```python
from build123d import *

# Parameters (mm, degrees)
F1_DEPTH     = 10.16
F5_R         = 1.4478
F6_DEPTH     = 25.4
F10_DEPTH    = 1.27
F11_T1_DEPTH = 22.6859947386
F11_T4_ANGLE = 28.0699881424
F11_T6_ANGLE = 28.0699881424


# Not quite as in the source:
# - a fillet or chamfer that OpenCascade refuses, or shapes differently, is made with other operations: its cross-section is extruded or revolved along the edge and cut away or added


with BuildPart() as f1:
    # F0 (on Top) → F1 (new body)
    with BuildSketch(Plane.XY):
        with BuildLine():
            ThreePointArc((0, 95.25), (-8.3015844967, 94.8875449932), (-16.5399889228, 93.8029384744))
            Line((-16.5399889228, 93.8029384744), (-15.6578561802, 88.8001150891))
            ThreePointArc((-15.6578561802, 88.8001150891), (-7.8588333236, 89.8268759269), (0, 90.17))
            Line((0, 90.17), (0, 95.25))
        make_face()
        with BuildLine():
            Line((15.6578561802, 88.8001150891), (16.5399889228, 93.8029384744))
            ThreePointArc((16.5399889228, 93.8029384744), (8.3015844967, 94.8875449932), (0, 95.25))
            Line((0, 95.25), (0, 90.17))
            ThreePointArc((0, 90.17), (7.8588333236, 89.8268759269), (15.6578561802, 88.8001150891))
        make_face()
    extrude(amount=F1_DEPTH)

    # F5 (on line) → F6 (cut)
    with BuildSketch(Plane(origin=(0, 95.25, 0), x_dir=(-1, 0, 0), z_dir=(0, 1, 0))):
        with Locations((-9.525, 5.08)):
            Circle(F5_R)
        with BuildLine():
            ThreePointArc((10.9728, 5.08), (9.525, 6.5278), (8.0772, 5.08))
            ThreePointArc((8.0772, 5.08), (9.525, 3.6322), (10.9728, 5.08))
        make_face()
    extrude(amount=-F6_DEPTH, mode=Mode.SUBTRACT)

    # F9 (on line) → F10 (cut, symmetric)
    with BuildSketch(Plane(origin=(0, 90.17, 0), x_dir=(-1, 0, 0), z_dir=(0, 1, 0))):
        Polygon((7.62, 8.3795567884), (5.715, 5.08), (7.62, 1.7804432116), (11.43, 1.7804432116), (13.335, 5.08), (11.43, 8.3795567884), align=None)
        Polygon((-11.43, 8.3795567884), (-13.335, 5.08), (-11.43, 1.7804432116), (-7.62, 1.7804432116), (-5.715, 5.08), (-7.62, 8.3795567884), align=None)
    extrude(amount=F10_DEPTH, both=True, mode=Mode.SUBTRACT)

    # F11: fillet of radius 2.54 on 4 edges, made by hand

    # F11_s2 → F11_t1 (cut)
    with BuildSketch(Plane.XY.offset(-6.2629973693)):
        with BuildLine():
            ThreePointArc((13.2190987409, 89.1957640725), (15.0767198196, 89.6478290697), (16.0928794122, 91.2672544357))
            Line((16.0928794122, 91.2672544357), (15.6578561802, 88.8001150891))
            ThreePointArc((15.6578561802, 88.8001150891), (14.4398326136, 89.0062926657), (13.2190987409, 89.1957640725))
        make_face()
        with BuildLine():
            ThreePointArc((-16.0928794122, 91.2672544357), (-15.0767198196, 89.6478290697), (-13.2190987409, 89.1957640725))
            ThreePointArc((-13.2190987409, 89.1957640725), (-14.4398326136, 89.0062926657), (-15.6578561802, 88.8001150891))
            Line((-15.6578561802, 88.8001150891), (-16.0928794122, 91.2672544357))
        make_face()
    extrude(amount=F11_T1_DEPTH, mode=Mode.SUBTRACT)

    # F11_s3 → F11_t4 (revolve, cut)
    with BuildSketch(Plane(origin=(0, 0, 0), x_dir=(0, 0, 1), z_dir=(-0.9701477887, -0.24251447, 0))):
        with BuildLine():
            ThreePointArc((7.62, 90.17), (9.4160512242, 90.9139487758), (10.16, 92.71))
            Line((10.16, 92.71), (10.16, 90.17))
            Line((10.16, 90.17), (7.62, 90.17))
        make_face()
    revolve(axis=Axis((0, 0, 10.16), (0, 0, -1)), revolution_arc=F11_T4_ANGLE, mode=Mode.SUBTRACT)

    # F11_s5 → F11_t6 (revolve, cut)
    with BuildSketch(Plane(origin=(0, 0, 0), x_dir=(0, 0, 1), z_dir=(-0.9701477887, -0.24251447, 0))):
        with BuildLine():
            ThreePointArc((2.54, 90.17), (0.7439487758, 90.9139487758), (0, 92.71))
            Line((0, 92.71), (0, 90.17))
            Line((0, 90.17), (2.54, 90.17))
        make_face()
    revolve(axis=Axis((0, 0, 0), (0, 0, -1)), revolution_arc=F11_T6_ANGLE, mode=Mode.SUBTRACT)


solid = f1.part
```
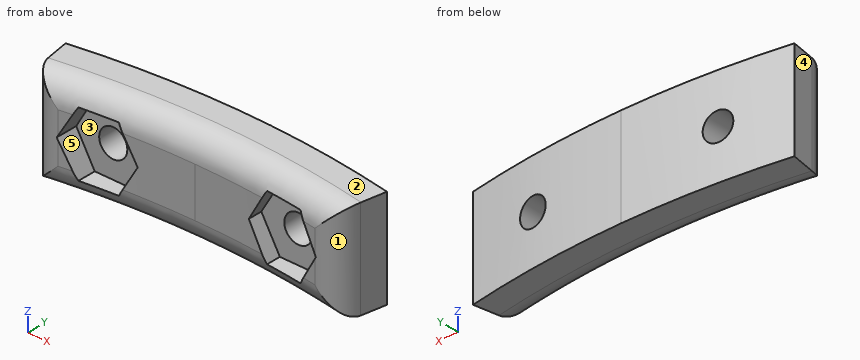
Geometry: final body of the model. Coordinates: model frame, mm. Face numbers are marked on the shaded views. A direction names the side the tool comes from. Give positions to 0.01 mm unless a question says otherwise; leave off trailing zeros. Loops run counter-clockwise (first coordinate to the right, second up) from the corner with the lowest first, then second, coordinate; pieces in that order, holes last. Notation, with made-up numbers: (68, -18) - (97, -18) arc R9 cw to (97, -9) - close; hole circle Ø10 at (73, 40). An arc over 180 degrees is marked (long way). Answer as CSV lines item,"result". Start each with the question number.
(1) Section query A-A (z = 2.25). Output: boundary loops of the cut face in (x, y), and give its area (3 significant figures).
(2) Section query B-B (y = 91.75). Give the number of separate pieces and of enclosed holes in the cut face, and give its area (3 significant figures).
(3) Mould query, pull axis Z, two halves, no side actions, for the marked faces 1, 2 and 3. Classes: +Z half, -Z half, draft (parallel to the pull), parting line (faces both ways), or undercut.
(4) Pin query (flat end, axial travel): P1, Ø4.5, axis at x = -9.525, z = 5.08, coming from the +Y side; P2, Ø0.9, axis at x = 9, y = 91, coming from the +Z side; P3, Ø2, axis at x = 9.5, y = 90.5, coming from the -Z side; P4, Ø2, axis at x = 9.5, z = 5, coming from the -Y side. Return the tip coordinate at first contact, or that it passes through.
(5) Ray query, line 1 along X through (y, z) = (92.65, 5.08); line 2 along X through (y, z) = (93.35, 5.08); line 3 along Z through (x, y) = (-10.5, 92.75). Return the intervals inside material, ascending. Write a range as [from, to].
(6) Reachability of the marked faces 4 and 5 from +Z, -Z, +X, -X, +Y, -Y: full face, straight path, thin tool, end or side. Return the list, or none.
Worked answers:
1,outline,"(-16.54, 93.8) - (-16.09, 91.27) arc R2.54 ccw to (-13.5, 89.17) arc R90.19 cw to (-11.7, 89.42) - (-11.7, 91.44) - (-7.35, 91.44) - (-7.35, 89.89) arc R90.19 cw to (7.35, 89.89) - (7.35, 91.44) - (11.7, 91.44) - (11.7, 89.42) arc R90.19 cw to (13.5, 89.17) arc R2.54 ccw to (16.09, 91.27) - (16.54, 93.8) arc R95.25 ccw to start"
1,area,"146 mm^2"
2,separate pieces,"1"
2,enclosed holes,"2"
2,area,"310 mm^2"
3,face 1,"draft"
3,face 2,"+Z half"
3,face 3,"undercut"
4,P1,"stops at y = 94.97"
4,P2,"stops at z = 10.03"
4,P3,"stops at z = 0.1"
4,P4,"passes through"
5,line 1,"x = [-16.34, -10.97], [-8.08, 8.08], [10.97, 16.34]"
5,line 2,"x = [-16.46, -10.97], [-8.08, 8.08], [10.97, 16.46]"
5,line 3,"z = [0, 4.01], [6.15, 10.16]"
6,face 4,"+Z, -Z, -X, -Y"
6,face 5,"-Y"
